from build123d import *

# Parameters (mm, degrees)
F1_DEPTH = 76.2
F3_D     = 15.875
F4_SIZE  = 3.175
F6_D     = 9.525


with BuildPart() as f1:
    # F0 (on Front) → F1 (new body)
    with BuildSketch(Plane.XZ):
        with BuildLine():
            Line((-31.750001, 38.1), (-38.1, 38.1))
            Line((-38.1, 38.1), (-38.1, -38.1))
            Line((-38.1, -38.1), (38.1, -38.1))
            Line((38.1, -38.1), (38.1, 38.1))
            Line((38.1, 38.1), (31.75, 38.1))
            Line((31.75, 38.1), (31.75, -25.400001))
            ThreePointArc((31.75, -25.400001), (29.890128, -29.890129), (25.4, -31.750001))
            Line((25.4, -31.750001), (-25.400001, -31.750001))
            ThreePointArc((-25.400001, -31.750001), (-29.890129, -29.890129), (-31.750001, -25.400001))
            Line((-31.750001, -25.400001), (-31.750001, 38.1))
        make_face()
    extrude(amount=F1_DEPTH)

    # F3 (through all)
    with Locations(Plane.YZ.offset(38.1)):
        with Locations((-38.1, 19.05)):
            Hole(F3_D / 2)

    # F4
    f4_edges = [f1.edges().sort_by_distance(p)[0] for p in [
        (-34.925001, 0, 38.1),
        (34.925, 0, 38.1),
        (34.925, -76.2, 38.1),
        (-34.925001, -76.2, 38.1),
    ]]
    chamfer(f4_edges, length=F4_SIZE)

    # F6 (through all)
    with Locations(Plane(origin=(0, 0, -38.1), x_dir=(1, 0, 0), z_dir=(0, 0, -1))):
        with Locations((-19.05, 57.15), (19.05, 57.15), (-19.05, 19.05), (19.05, 19.05)):
            Hole(F6_D / 2)


solid = f1.part
Can you work these out from the model? Positions are in its coordinate system, mm. A direction names the side the tool comes from. Give positions to 0.01 mm unless a question says otherwise; leave off trailing zeros. Loops run counter-clockwise (first coordinate to the right, second up) from the corner with the lowest first, then second, coordinate; pieces in that order, holes last. Notation, with made-up numbers: M 68.5,-31 L 77.5,-31 A10 ccw 77.5,-17 Z; hole C -6,13 d2. An arc over 180 degrees is marked long. One line per item, written item: value.
1) I'm going to push a flat-ended pin straight in: pin 1 (6 mm diameter, centred on x = -8.5, y = -30.5, fed in from +Z). Where does the tip first touch, or does it pass through?
Geometry check:
pin 1: stops at z = -31.75
2) Thinking about a two-plate mould opening in Y: for faces 3 (the face through (34.969, -1.61, 36.535)), 4 (the face through (-1, -38, -38.1)), 5 (the face through (14.507, -58.581, -34.881)), which applies, +Y half, -Y half, draft (parallel to the pull), parting line (faces both ways), or undercut?
Geometry check:
face 3: +Y half
face 4: draft
face 5: undercut
3) On a 3-axis mill with a long thin cutter (end or side, diameter ignored), from which of +Z, -Z, +X, -X, +Y, -Y can I reach the whole of each face in a straight line? I mean faces 1 (the face through (-34.881, -1.565, 36.49)), 2 (the face through (-29.84, -37.57, -29.94)). Say none if no direction works.
Geometry check:
face 1: +Z, +X, -X, +Y
face 2: +Z, +Y, -Y
4) Imagine slicing it at D-D on y = -27.5. Write out the boundary of the cut face in (x, z).
Geometry check:
outline: M -38.1,-38.1 L 38.1,-38.1 L 38.1,38.1 L 31.75,38.1 L 31.75,-25.4 A6.35 cw 25.4,-31.75 L -25.4,-31.75 A6.35 cw -31.75,-25.4 L -31.75,38.1 L -38.1,38.1 Z
5) Imagine slicing it at B-B on z = 31. Write out the boundary of the cut face in (x, y).
Geometry check:
outline: M -38.1,-76.2 L -31.75,-76.2 L -31.75,0 L -38.1,0 Z; M 31.75,-76.2 L 38.1,-76.2 L 38.1,0 L 31.75,0 Z
6) Please list where these lines run through material, in increasing order: line 1 (Y direction, x = 19, z = -34); line 2 (X direction, y = -27, z = 22.5); line 3 (Z direction, x = 36, y = -38).
Geometry check:
line 1: y = -76.2 to -61.91, -52.39 to -23.81, -14.29 to 0
line 2: x = -38.1 to -31.75, 31.75 to 38.1
line 3: z = -38.1 to 11.11, 26.99 to 38.1
7) Imagine slicing it at C-C on x = -19.05. Write out the boundary of the cut face in (y, z).
Geometry check:
outline: M -76.2,-38.1 L -61.91,-38.1 L -61.91,-31.75 L -76.2,-31.75 Z; M -52.39,-38.1 L -23.81,-38.1 L -23.81,-31.75 L -52.39,-31.75 Z; M -14.29,-38.1 L 0,-38.1 L 0,-31.75 L -14.29,-31.75 Z
8) Imagine slicing it at A-A on y = -38.1. Write out the boundary of the cut face in (x, z), and give its area (3 significant figures).
Geometry check:
outline: M -38.1,-38.1 L 38.1,-38.1 L 38.1,11.11 L 31.75,11.11 L 31.75,-25.4 A6.35 cw 25.4,-31.75 L -25.4,-31.75 A6.35 cw -31.75,-25.4 L -31.75,11.11 L -38.1,11.11 Z; M -38.1,26.99 L -31.75,26.99 L -31.75,38.1 L -38.1,38.1 Z; M 31.75,26.99 L 38.1,26.99 L 38.1,38.1 L 31.75,38.1 Z
area: 1,190 mm²
